from build123d import *

# Parameters (mm, degrees)
BOSS_EXTRUDE1_DEPTH = 12.7
SKETCH2_R           = 0.6
CUT_EXTRUDE1_DEPTH  = 3.175
FILLET1_R           = 2.54


with BuildPart() as part:
    # Sketch1 → Boss-Extrude1 (new body)
    with BuildSketch(Plane.XY):
        with BuildLine():
            Line((0, 16.475869837), (0, -11.718130163))
            ThreePointArc((0, -11.718130163), (0.371974388, -12.616155775), (1.27, -12.988130163))
            Line((1.27, -12.988130163), (13.97, -12.988130163))
            Line((13.97, -12.988130163), (13.97, -16.163130163))
            Line((13.97, -16.163130163), (1.27, -16.163130163))
            ThreePointArc((1.27, -16.163130163), (-1.873089642, -14.861219805), (-3.175, -11.718130163))
            Line((-3.175, -11.718130163), (-3.175, 16.475869837))
            Line((-3.175, 16.475869837), (0, 16.475869837))
        make_face()
    extrude(amount=BOSS_EXTRUDE1_DEPTH)

    # Sketch2 → Cut-Extrude1 (cut)
    with BuildSketch(Plane.ZY.offset(3.175)):
        with Locations(Location((6.380886644, 0.665885837, 0), (0, 0, 270))):
            Circle(SKETCH2_R)
        with Locations(Location((6.35, 4.665877837, 0), (0, 0, 270))):
            Circle(SKETCH2_R)
        with Locations(Location((6.35, 8.665869837, 0), (0, 0, 270))):
            Circle(SKETCH2_R)
        with Locations(Location((6.35, 12.665869837, 0), (0, 0, 270))):
            Circle(SKETCH2_R)
    extrude(amount=-CUT_EXTRUDE1_DEPTH, mode=Mode.SUBTRACT)

    # Fillet1
    fillet1_edges = [part.edges().sort_by_distance(p)[0] for p in [
        (-1.5875, 16.475869837, 0),
        (13.97, -14.575630163, 12.7),
        (-1.5875, 16.475869837, 12.7),
        (13.97, -14.575630163, 0),
    ]]
    fillet(fillet1_edges, radius=FILLET1_R)


solid = part.part
Could you check a few things on this model? Use its own coordinates, in mm. A direction names the side the tool comes from. Give positions to 0.01 mm unless a question says otherwise; leave off trailing zeros. Order: outer loops, then holes, each group sorted by start corner. A loop starts at its lowest first (then second) coordinate and runs counter-clockwise, first axis right, second up. Notation, with made-up numbers: (83, 71) -> (132, 71) arc R11 cw to (132, 91) -> close; hole circle Ø9 at (6.25, 37). An arc over 180 degrees is marked (long way). Answer in a Markdown table with one row per item. Add a question column.
Item 1: Imagine slicing it at D-D (y = -9.5). List the corners of the cut face in (x, z) for me (3 decimals).
Item 2: Imagine slicing it at A-A (y = 0.5). List the corners of the cut face in (x, z) for me (1 decimal), and give its area (3 significant figures).
Item 3: We'd pull the mould along Z, two halves only. Please class faces 3 (the flat face through (8, -16.163, 6)), 4 (the cylindrical face through (-1.57, 15.75, 0.76)), 5 (the cylindrical face through (-1.61, 0.744, 6.976)): pulls with the +Z half, pulls with the -Z half, needs draft (parallel to the pull), parting line crosses it, or undercut.
Item 4: For faces 1 (the flat face through (0, 3, 6)), 2 (the cylindrical face through (-1.838, -14.896, 6.261)), which set-ups out of +Z, -Z, +X, -X, +Y, -Y let a thin tool reach every point of the face, with its end or its side?
Item 5: I'm going to push flat-ended pins straight in: P1, Ø4, axis at y = 7.5, z = 8, coming from the +X side; P2, Ø5, axis at x = 10.5, z = 8.5, coming from the +Y side. Where does each tip first touch, or does it pass through?
Item 6: Imagine slicing it at C-C (x = -2). List the corners of the cut face in (y, z) for me, and give its area (3 significant figures).
Item 7: Imagine slicing it at B-B (z = 5.25). List the corners of the cut face in (x, y) for me (3 decimals).
Item 8: Please list where these lines run through material, in increasing order: probe 1 along Y at (x, z) = (8.25, 9); probe 2 along X at (y, z) = (7.5, 10.5) (3 decimals); probe 3 along Y at (x, z) = (-0.75, 5).
Result:
| question | item | result |
|---|---|---|
| 1 | outline | (-3.175, 0) -> (0, 0) -> (0, 12.7) -> (-3.175, 12.7) -> close |
| 2 | outline | (-3.2, 0) -> (0, 0) -> (0, 5.8) -> (-3.2, 5.8) -> close; (-3.2, 7) -> (0, 7) -> (0, 12.7) -> (-3.2, 12.7) -> close |
| 2 | area | 36.7 mm2 |
| 3 | face 3 | needs draft |
| 3 | face 4 | pulls with the -Z half |
| 3 | face 5 | undercut |
| 4 | face 1 | +Z, -Z, +X, +Y |
| 4 | face 2 | +Z, -Z, -X, -Y |
| 5 | P1 | x = 0 |
| 5 | P2 | y = -12.99 |
| 6 | outline | (-14.73, 0) -> (13.94, 0) arc R2.54 ccw to (16.48, 2.54) -> (16.48, 10.16) arc R2.54 ccw to (13.94, 12.7) -> (-14.73, 12.7) -> close; hole circle Ø1.2 at (0.67, 6.38); hole circle Ø1.2 at (4.67, 6.35); hole circle Ø1.2 at (8.67, 6.35); hole circle Ø1.2 at (12.67, 6.35) |
| 6 | area | 389 mm2 |
| 7 | outline | (-3.175, -11.718) arc R4.445 ccw to (1.27, -16.163) -> (13.97, -16.163) -> (13.97, -12.988) -> (1.27, -12.988) arc R1.27 cw to (0, -11.718) -> (0, 16.476) -> (-3.175, 16.476) -> close |
| 8 | probe 1 | -16.16 to -12.99 |
| 8 | probe 2 | -3.175 to 0 |
| 8 | probe 3 | -15.68 to 16.48 |
